```python
from build123d import *

# Parameters (mm, degrees)
BOSS_EXTRUDE1_DEPTH = 10
SKETCH2_R           = 10
CUT_EXTRUDE1_DEPTH  = 10
BOSS_EXTRUDE2_DEPTH = 10
BOSS_EXTRUDE3_DEPTH = 10


with BuildPart() as part:
    # Sketch1 → Boss-Extrude1 (new body)
    with BuildSketch(Plane.XY):
        Polygon((-15.751690718, 35.056562454), (14.248309282, 35.056562454), (24.248309282, 25.056562454), (24.248309282, -14.943437546), (-25.751690718, -14.943437546), (-25.751690718, 25.056562454), align=None)
    extrude(amount=-BOSS_EXTRUDE1_DEPTH)

    # Sketch2 → Cut-Extrude1 (cut)
    with BuildSketch(Plane.XY):
        with Locations((-0.751690718, 20.056562454)):
            Circle(SKETCH2_R)
    extrude(amount=-CUT_EXTRUDE1_DEPTH, mode=Mode.SUBTRACT)

    # Sketch3 → Boss-Extrude2 (add)
    with BuildSketch(Plane(origin=(24.248309282, 0, 0), x_dir=(0, 0, -1), z_dir=(1, 0, 0))):
        Polygon((0, -14.943437546), (-25, -14.943437546), (-10, 5.056562454), (0, 5.056562454), align=None)
    extrude(amount=-BOSS_EXTRUDE2_DEPTH)

    # Sketch4 → Boss-Extrude3 (add)
    with BuildSketch(Plane.ZY.offset(25.751690718)):
        Polygon((0, -14.943437546), (25, -14.943437546), (10, 5.056562454), (0, 5.056562454), align=None)
    extrude(amount=-BOSS_EXTRUDE3_DEPTH)


solid = part.part
```
Geometry: final body of the model. Coordinates: model frame, mm. A direction names the side the tool comes from. Round coordinates to 2 decimals unless told otherwise and drop trailing zeros. Write each loop counter-clockwise with the first axis right and the second up, starting at its lowest first coordinate (ties: lowest second). Pieces come first, ordered by that corner, then holes. Notation, with made-up numbers: (-14.75, -32.75) -> (2.25, -32.75) arc R21 ccw to (2.25, -4.75) -> close; hole circle Ø6 at (9.5, 72.25). An arc over 180 degrees is marked (long way). Return JSON: item names as keys, results as strings.
Q1. Section C-C on z = -5.5. Return the cut outline in (x, y).
From the geometry:
{"outline": "(-25.75, -14.94) -> (24.25, -14.94) -> (24.25, 25.06) -> (14.25, 35.06) -> (-15.75, 35.06) -> (-25.75, 25.06) -> close; hole circle Ø20 at (-0.75, 20.06)"}
Q2. Set-up query: faces 5 (the flat face through (-15.752, -7, 10)), 6 (the flat face through (-25.752, 1, 3)), 7 (the flat face through (-21, 5.057, 5)). Return all of +Z, -Z, +X, -X, +Y, -Y with unobstructed straight access to the full face (end or side cutting, diameter ignored); none if empty.
From the geometry:
{"face 5": "+Z, +Y, -Y", "face 6": "+Z, -Z, -X, +Y, -Y", "face 7": "+Z, +X, -X, +Y"}
Q3. Mould query, pull axis X, two halves, no side actions, for faces 1 (the flat face through (24.248, 1, 3)), 2 (the flat face through (19, 5.057, 5)), 3 (the flat face through (-20.82, 29.99, -4.93)), 4 (the flat face through (14.248, -7, 10)). Classes: +X half, -X half, draft (parallel to the pull), parting line (faces both ways), or undercut.
From the geometry:
{"face 1": "+X half", "face 2": "draft", "face 3": "-X half", "face 4": "undercut"}
Q4. Ray query, line 1 (X direction, y = -4, z = 13); line 2 (Y direction, x = -16, z = 0.5); line 3 (Z direction, x = 11, y = 9). Return the intervals inside material, ascending.
From the geometry:
{"line 1": "-25.75 to -15.75, 14.25 to 24.25", "line 2": "-14.94 to 5.06", "line 3": "-10 to 0"}
Q5. Section D-D on y = 1.5. Return the cut outline in (x, z), and give its area (3 significant figures).
From the geometry:
{"outline": "(-25.75, -10) -> (24.25, -10) -> (24.25, 12.67) -> (14.25, 12.67) -> (14.25, 0) -> (-15.75, 0) -> (-15.75, 12.67) -> (-25.75, 12.67) -> close", "area": "753 mm2"}
Q6. First-contact query: pin 1 Ø5 at (x, z) = (-22, 7.5) entering from +Y; pin 2 Ø10 at (x, y) = (17, 19.5) entering from +Z; pin 3 Ø23 at (x, y) = (-0.75, 20.06) entering from -Z. Flat tips, straight axial feed; report the tip coordinate or a pass-through.
From the geometry:
{"pin 1": "y = 5.06", "pin 2": "z = 0", "pin 3": "z = -10"}
Q7. Section A-A on z = 6.5. Return the cut outline in (x, y).
From the geometry:
{"outline": "(-25.75, -14.94) -> (-15.75, -14.94) -> (-15.75, 5.06) -> (-25.75, 5.06) -> close; (14.25, -14.94) -> (24.25, -14.94) -> (24.25, 5.06) -> (14.25, 5.06) -> close"}
Q8. Section B-B on x = -3. Return the cut outline in (y, z), and give its area (3 significant figures).
From the geometry:
{"outline": "(-14.94, -10) -> (10.31, -10) -> (10.31, 0) -> (-14.94, 0) -> close; (29.8, -10) -> (35.06, -10) -> (35.06, 0) -> (29.8, 0) -> close", "area": "305 mm2"}
